```python
from build123d import *

# Parameters (mm, degrees)
CYLINDER002_R           = 1.5
CYLINDER002_DEPTH       = 20
CYLINDER002_PITCH_ANGLE = 90
CYLINDER001_R           = 2.5
CYLINDER001_DEPTH       = 30
BOX_W                   = 2.4
BOX_H                   = 5.5
BOX_DEPTH               = 20
FILLET_1_R              = 1.5
FILLET_2_R              = 1


with BuildPart() as clone_of_bolt:
    # Cylinder002 → Cylinder002 (new body)
    with BuildSketch(Plane.XY):
        Circle(CYLINDER002_R)
    extrude(amount=CYLINDER002_DEPTH)


with BuildPart() as clone_of_bolt_1:
    # Cylinder002 pitch: moved
    add(clone_of_bolt.part.rotate(Axis((0, 0, 0), (0, 1, 0)), CYLINDER002_PITCH_ANGLE))


with BuildPart() as clone_of_bolt_2:
    # Cylinder002 placement: moved
    add(clone_of_bolt_1.part.moved(Location((0, 0, 3.5))))


with BuildPart() as clone_of_nemashaft:
    # Cylinder001 → Cylinder001 (new body)
    with BuildSketch(Plane.XY.offset(-8)):
        Circle(CYLINDER001_R)
    extrude(amount=CYLINDER001_DEPTH)


with BuildPart() as innercavity:
    # Box → Box (new body)
    with BuildSketch(Plane(origin=(4, -2.75, -13), x_dir=(1, 0, 0), z_dir=(0, 0, 1))):
        with Locations((1.2, 2.75)):
            Rectangle(BOX_W, BOX_H)
    extrude(amount=BOX_DEPTH)

    # Fusion: union Clone of Bolt, Clone of NEMAShaft
    add(clone_of_bolt_2.part)
    add(clone_of_nemashaft.part)


with BuildPart() as innercavitycut:
    # Sketch001 → Revolution (revolve)
    with BuildSketch(Plane.XZ):
        Polygon((0, 16), (7, 16), (7, 13.5), (5.5, 12), (5.5, 8), (10, 6.362134), (10, 0), (0, 0), align=None)
    revolve(axis=Axis((0, 0, 0), (0, 0, 1)))

    # Fillet 1
    fillet_1_edges = [innercavitycut.edges().sort_by_distance(p)[0] for p in [
        (-10, 0, 6.362134),
    ]]
    fillet(fillet_1_edges, radius=FILLET_1_R)

    # Fillet 2
    fillet_2_edges = [innercavitycut.edges().sort_by_distance(p)[0] for p in [
        (-7, 0, 13.5),
    ]]
    fillet(fillet_2_edges, radius=FILLET_2_R)

    # Cut: cut InnerCavity
    add(innercavity.part, mode=Mode.SUBTRACT)


solid = innercavitycut.part
```
Work out the finished part from the listing and answer in its coordinate system (mm). A direction names the side the tool comes from. Give positions to 0.01 mm unless a question says otherwise; leave off trailing zeros. Loops run counter-clockwise (first coordinate to the right, second up) from the corner with the lowest first, then second, coordinate; pieces in that order, holes last. Notation, with made-up numbers: (2, 74) -> (33, 74) arc R25 ccw to (33, 100) -> close; hole circle Ø9 at (18.25, 55.5). An arc over 180 degrees is marked (long way). Use CSV: the item, a comma, the result in double quotes.
1. Straight lines are drawn through the part: line 1 (Z direction, x = 2.65, y = 0); line 2 (Z direction, x = 9, y = 0); line 3 (X direction, y = 2, z = 6.25). For each, find the intervals that lie inside material, in ascending order.
Found:
line 1,"0 to 2, 5 to 16"
line 2,"0 to 2, 5 to 6.73"
line 3,"-9.46 to -1.5, 1.5 to 4, 6.4 to 9.46"
2. The mould has two halves that part along Z. Classify faces 6 (the cylindrical face through (3.21, 1.01, 4.61)), 7 (the conical face through (-1.24, -5.58, 7.92)), 8 (the flat face through (0, -3, 16)), 9 (the flat face through (5, 2.75, 3)): +Z half, -Z half, draft (parallel to the pull), parting line (faces both ways), or undercut.
Found:
face 6,"undercut"
face 7,"undercut"
face 8,"+Z half"
face 9,"draft"
3. Flat-ended cylindrical pins translate along their axes: pin 1 Ø1 at (y, z) = (2, 7) entering from +X; pin 2 Ø0.7 at (x, z) = (5, 2.5) entering from -Y; pin 3 Ø4 at (y, z) = (7, 4) entering from -X; pin 4 Ø3 at (x, y) = (0, 0) entering from +Z. Find the tip coordinate at first contact, or state that the pin passes through.
Found:
pin 1,"x = 9.21"
pin 2,"y = -8.85"
pin 3,"x = -8.66"
pin 4,"through"
4. The part is cut by section A-A (y = 0). State how many separate pieces and enclosed holes the cut face has, then the cut area to 3 significant figures.
Found:
separate pieces,"4"
enclosed holes,"0"
area,"138 mm^2"
5. The part is cut by section B-B (z = 3.5). Write down the section's boundary in (x, y), then the cut area to 3 significant figures.
Found:
outline,"(2, -1.5) arc R2.5 cw (long way) to (2, 1.5) -> (4, 1.5) -> (4, 2.75) -> (6.4, 2.75) -> (6.4, 1.5) -> (9.89, 1.5) arc R10 ccw (long way) to (9.89, -1.5) -> (6.4, -1.5) -> (6.4, -2.75) -> (4, -2.75) -> (4, -1.5) -> close"
area,"266 mm^2"
6. A tool of negligible diameter and unlimited length cuts with its end or side. For faces 1 (the cylindrical face through (-2.5, 0.1, 7.9)), 2 (the cylindrical face through (-1.19, -5.37, 9.97)), 3 (the cylindrical face through (8.175, -0.575, 2.114)), 4 (the flat face through (4, -1, 2)), 5 (the cylindrical face through (6.466, -2.681, 14.943)), from which of +Z, -Z, +X, -X, +Y, -Y can it reach the whole face along a straight path? Write none if from no direction.
Found:
face 1,"+Z, -Z"
face 2,"none"
face 3,"+X"
face 4,"-Z"
face 5,"+Z"
